Part print with two shaded views. Sizes in mm from the minimum x, y, z corner. Round coordinates to 2 decimals unless told otherwise and drop trailing zeros. Order: outer loops, then holes, each group sorted by start corner. A loop starts at its lowest first (then second) coordinate and runs counter-clockwise, first axis right, second up. Notation, with made-up numbers: M 51.5,36.5 L 80.5,36.5 A7 ccw 80.5,44.5 Z; hole C 74.25,59.25 d2. An arc over 180 degrees is marked long. One line per question, with ' | ' between items. Start each with the question number.
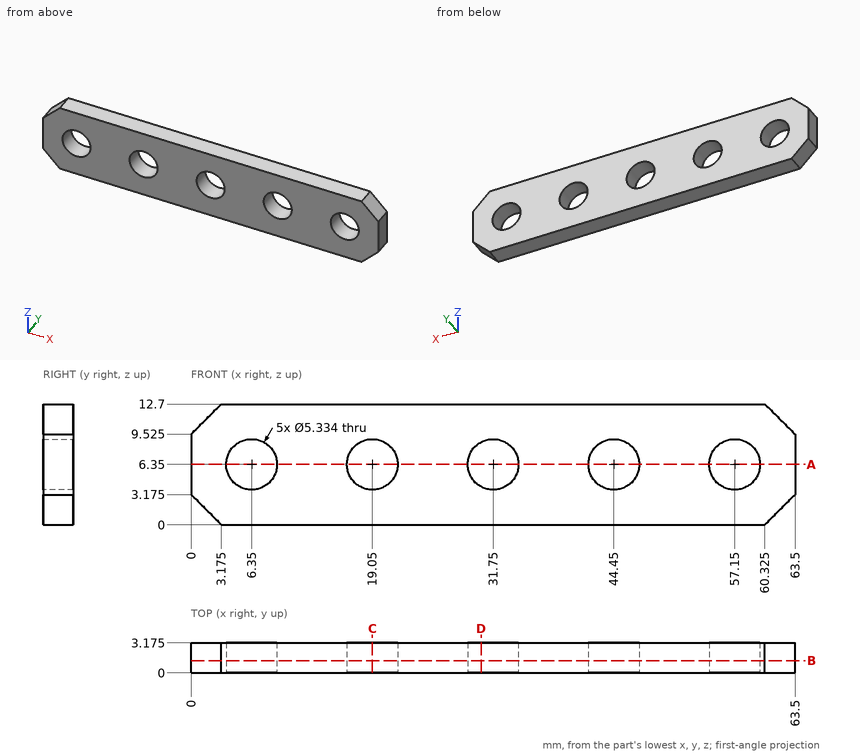
Item 1: Wall check: line 1 along X through (y, z) = (0.75, 6.35); line 2 along X through (y, z) = (2.35, 5.5); line 3 along Z through (x, y) = (6.5, 2.8). Give the ranges that are in metal, low to high. Write a range as [from, to].
Item 2: Cut at D-D on x = 30.5. Write the cut outline in (y, z) (3 decimals).
Item 3: Cut at A-A on z = 6.35. Write the cut outline in (x, y) (3 decimals).
Item 4: Cut at C-C on x = 19.05. Write the cut outline in (y, z) (3 decimals).
Item 5: Flat gauge pin, fed straight in: pin 1 (7 mm diameter, centred on x = 6.35, z = 6.35, fed in from -Y). Where does the tip first touch, or does it go through?
Item 6: Cut at B-B on y = 1.3. Write the cut outline in (x, z) (3 decimals).
Results found:
1) line 1: x = [0, 3.68], [9.02, 16.38], [21.72, 29.08], [34.42, 41.78], [47.12, 54.48], [59.82, 63.5] | line 2: x = [0, 3.82], [8.88, 16.52], [21.58, 29.22], [34.28, 41.92], [46.98, 54.62], [59.68, 63.5] | line 3: z = [0, 3.69], [9.01, 12.7]
2) outline: M 0,0 L 3.175,0 L 3.175,3.994 L 0,3.994 Z; M 0,8.706 L 3.175,8.706 L 3.175,12.7 L 0,12.7 Z
3) outline: M 0,0 L 3.683,0 L 3.683,3.175 L 0,3.175 Z; M 9.017,0 L 16.383,0 L 16.383,3.175 L 9.017,3.175 Z; M 21.717,0 L 29.083,0 L 29.083,3.175 L 21.717,3.175 Z; M 34.417,0 L 41.783,0 L 41.783,3.175 L 34.417,3.175 Z; M 47.117,0 L 54.483,0 L 54.483,3.175 L 47.117,3.175 Z; M 59.817,0 L 63.5,0 L 63.5,3.175 L 59.817,3.175 Z
4) outline: M 0,0 L 3.175,0 L 3.175,3.683 L 0,3.683 Z; M 0,9.017 L 3.175,9.017 L 3.175,12.7 L 0,12.7 Z
5) pin 1: stops at y = 0
6) outline: M 0,3.175 L 3.175,0 L 60.325,0 L 63.5,3.175 L 63.5,9.525 L 60.325,12.7 L 3.175,12.7 L 0,9.525 Z; hole C 6.35,6.35 d5.334; hole C 19.05,6.35 d5.334; hole C 31.75,6.35 d5.334; hole C 44.45,6.35 d5.334; hole C 57.15,6.35 d5.334
